For this review, take the finished solid that the model builds, in its own axes (mm). Face numbers are marked on the shaded views. A direction names the side the tool comes from. Round coordinates to 2 decimals unless told otherwise and drop trailing zeros. One line per item, written item: value. Start each with the question number.
Q1. For probe 1 along X at (y, z) = (-1, 5); probe 2 along Z at (x, y) = (5.25, -1.25); probe 3 along X at (y, z) = (-2.25, -7.25), list the stretches that pass through material, from the lowest coordinate up.
Q2. Add section A-A on z = -0.25. Give the number of separate pieces and of enclosed holes in the cut face, and give its area (3 significant figures).
Q3. Clearance check with flat-ended pins moving along their axes: pin 1 Ø5 at (y, z) = (1, 4.5) entering from +X; pin 2 Ø2 at (y, z) = (-1, 0) entering from -X; pin 3 Ø3 at (x, y) = (6.5, -0.5) entering from +Z; pin 4 Ø5 at (x, y) = (4, -3.5) entering from -Z. State where each tip first meets the part, or that it passes through.
Q4. Mouldability with a two-part tool opening along Z and no side actions: class the marked faces 3, 4 and 5 as +Z half, -Z half, draft (parallel to the pull), parting line (faces both ways), or undercut.
Q5. Tool access review of the marked faces 1 and 2: name each direction out of +Z, -Z, +X, -X, +Y, -Y from which nothing blocks a thin tool from reaching the whole face with its end or side.
```python
from build123d import *

# Parameters (mm, degrees)
BASE_DEPTH        = 3
BASE_DEPTH_BACK   = 7
SKETCH1_R         = 10
SKETCH2_R         = 1.6
HOLE1_DEPTH       = 19.934353276
HOLE1MIRROR_COUNT = 2
SKETCH3_R         = 1.6
HOLE2_DEPTH       = 19.445737601
HOLE2MIRROR_COUNT = 2
SKETCH4_R         = 1.6
HOLE3_DEPTH       = 19.389503466
HOLE3MIRROR_COUNT = 2
FILLET1_R         = 5


with BuildPart() as part:
    # Sketch1 → base (new, two sides: drawn at the far end of the back side and taken through both)
    with BuildSketch(Plane(origin=(0, 0, 0), x_dir=(1, 0, 0), z_dir=(0, 1, 0)).offset(-BASE_DEPTH_BACK)):
        with Locations(Location((0, 0, 0), (0, 0, 270))):
            Circle(SKETCH1_R)
    extrude(amount=BASE_DEPTH + BASE_DEPTH_BACK)

    # Sketch2 → hole1 (cut, through all)
    with BuildSketch(Plane(origin=(2.670502563, -1.093066116, 2.770130417), x_dir=(-0.6558691872850446, 0.22429081675253856, 0.7207837669443827), z_dir=(-0.6676256406563905, 0.27326652891267483, -0.692532604369038))):
        with Locations(Location((0, 0, 0), (0, 0, 346.516491398))):
            Circle(SKETCH2_R)
    hole1 = extrude(amount=-HOLE1_DEPTH, mode=Mode.SUBTRACT)

    # hole1mirror: hole1 ×2 about axis
    hole1mirror_axis = Axis((0, 5.5, 0), (0, -1, 0))
    for i in range(1, HOLE1MIRROR_COUNT):
        add(hole1.rotate(hole1mirror_axis, i * 360 / HOLE1MIRROR_COUNT), mode=Mode.SUBTRACT)

    # Sketch3 → hole2 (cut, through all)
    with BuildSketch(Plane(origin=(-0.941672921, -1.236067977, 3.685836142), x_dir=(-0.9718935871364875, 0.07382318789513377, -0.22354639834264944), z_dir=(0.23541823021467095, 0.3090169943749464, -0.921459035481267))):
        with Locations(Location((0, 0, 0), (0, 0, 90.062171088))):
            Circle(SKETCH3_R)
    hole2 = extrude(amount=-HOLE2_DEPTH, mode=Mode.SUBTRACT)

    # hole2mirror: hole2 ×2 about axis
    hole2mirror_axis = Axis((0, 5.5, 0), (0, -1, 0))
    for i in range(1, HOLE2MIRROR_COUNT):
        add(hole2.rotate(hole2mirror_axis, i * 360 / HOLE2MIRROR_COUNT), mode=Mode.SUBTRACT)

    # Sketch4 → hole3 (cut, through all)
    with BuildSketch(Plane(origin=(-3.717841, -1.236067977, 0.806098168), x_dir=(-0.19123247894507908, -0.06357892752956036, -0.979483465389136), z_dir=(0.9294602499075393, 0.30901699437494623, -0.20152454200243008))):
        with Locations(Location((0, 0, 0), (0, 0, 90))):
            Circle(SKETCH4_R)
    hole3 = extrude(amount=-HOLE3_DEPTH, mode=Mode.SUBTRACT)

    # hole3mirror: hole3 ×2 about axis
    hole3mirror_axis = Axis((0, 5.5, 0), (0, -1, 0))
    for i in range(1, HOLE3MIRROR_COUNT):
        add(hole3.rotate(hole3mirror_axis, i * 360 / HOLE3MIRROR_COUNT), mode=Mode.SUBTRACT)

    # Fillet1
    # the kernel refuses this fillet: 5 mm, written as the material it takes off along each edge
    with BuildSketch(Plane(origin=(0, -7, 0), x_dir=(0, 0, 1), z_dir=(-1, 0, 0))) as fillet1_piece_1:
        with BuildLine():
            CenterArc((10 - FILLET1_R, FILLET1_R), FILLET1_R, 270, 90)
            Line((10 - FILLET1_R, 0), (10, 0))
            Line((10, 0), (10, FILLET1_R))
        make_face()
    revolve(axis=Axis((0, -7, 0), (0, 1, 0)), mode=Mode.SUBTRACT)
    with BuildSketch(Plane(origin=(0, 3, 0), x_dir=(0, 0, 1), z_dir=(-1, 0, 0))) as fillet1_piece_2:
        with BuildLine():
            CenterArc((10 - FILLET1_R, -FILLET1_R), FILLET1_R, 0, 90)
            Line((10 - FILLET1_R, 0), (10, 0))
            Line((10, 0), (10, -FILLET1_R))
        make_face()
    revolve(axis=Axis((0, 3, 0), (0, 1, 0)), mode=Mode.SUBTRACT)


solid = part.part
```
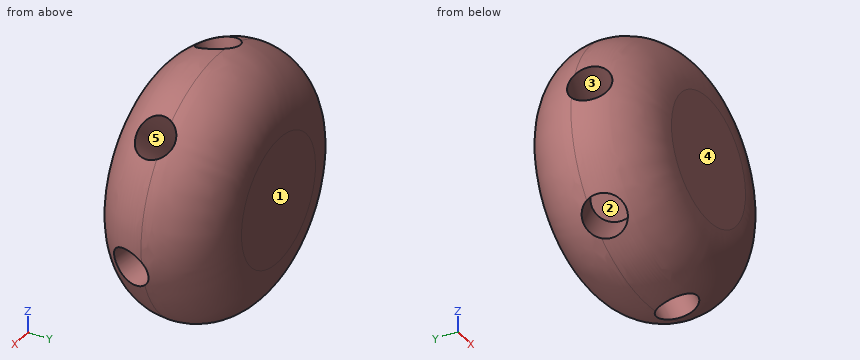
Result set:
1. probe 1: x = -8.54 to -2.73, 0.28 to 2.73, 6.27 to 8.54
1. probe 2: z = -8.44 to -2.67, 0.46 to 3.22, 7.01 to 8.44
1. probe 3: x = -4.78 to 0.2, 3.48 to 6.88
2. separate pieces: 1
2. enclosed holes: 2
2. area: 163 mm^2
3. pin 1: stops at x = 9.46
3. pin 2: stops at x = -10
3. pin 3: stops at z = 8.49
3. pin 4: stops at z = -9.68
4. face 3: undercut
4. face 4: draft
4. face 5: undercut
5. face 1: +Z, -Z, +X, -X, +Y
5. face 2: none
